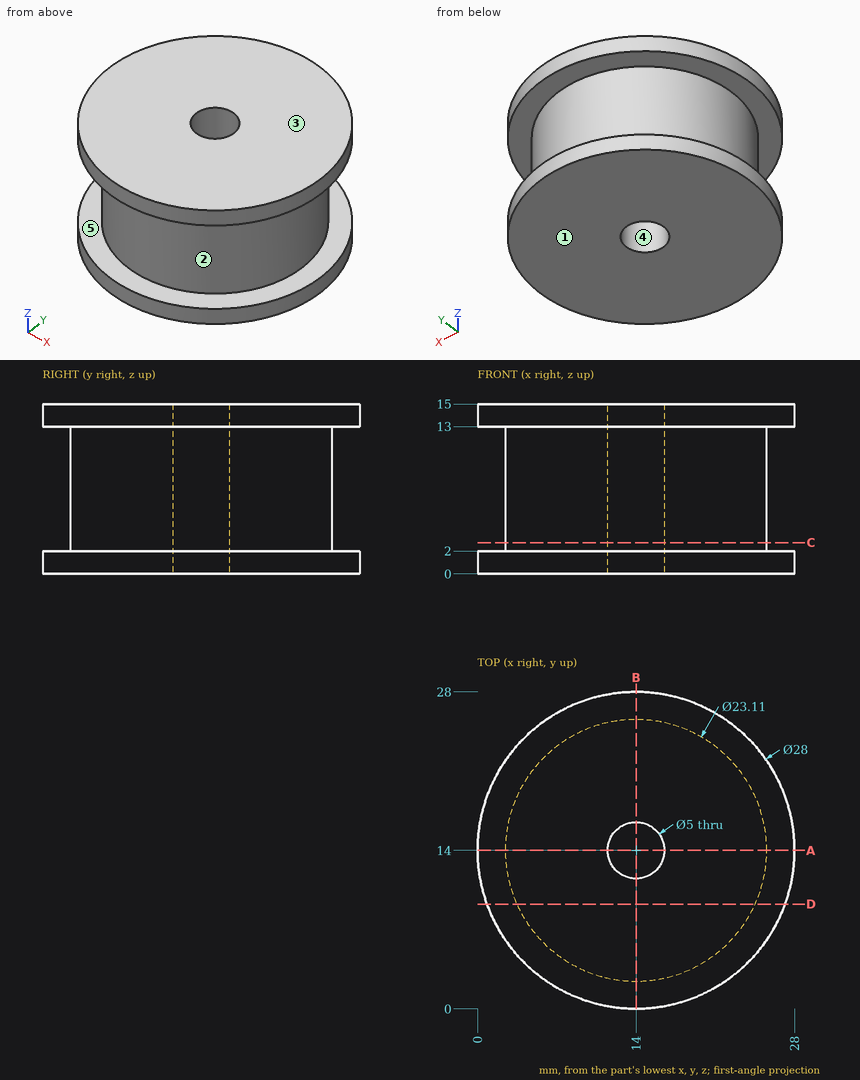
Design review of the part shown in the three views and the two pictorial views. Dimensions are in mm from the part's minimum x, y and z. A direction names the side the tool comes from. Give positions to 0.01 mm unless a question says otherwise; leave off trailing zeros. Write each loop counter-clockwise with the first axis right and the second up, starting at its lowest first coordinate (ties: lowest second). Pieces come first, ordered by that corner, then holes. Notation, with made-up numbers: M -25.75,-38 L 24.25,-38 A10 cw 24.25,-34 Z; hole C 14.25,-18 d11. An arc over 180 degrees is marked long. One line per item, written item: value.
1) Take a section at C-C, the plane z = 2.75. Write out the cut boundary in (x, y) (3 decimals), then the cut area to 3 significant figures.
Results are:
outline: C 14,14 d23.11; hole C 14,14 d5
area: 400 mm²
2) For P1, Ø6, axis at x = 21.5, z = 2.5, coming from the -Y side; P2, Ø3, axis at x = 14, y = 14, coming from the -Z side; P3, Ø1, axis at y = 15.5, z = 13, coming from the -X side; P4, Ø2, axis at y = 13, z = 8, coming from the +X side (3 decimals), all flat-tipped, find the tip position at first contact; note any pin that passes through.
Results are:
P1: stops at y = 0.76
P2: passes through
P3: stops at x = 0.04
P4: stops at x = 25.555
3) For the marked faces 4 and 5, list the 3-axis set-ups (+Z, -Z, +X, -X, +Y, -Y) from which the entire face can be reached by the end or side of a thin tool; tool diameter is ignored.
Results are:
face 4: +Z, -Z
face 5: none
4) The part is to be moulded in two halves that separate along Z. For the marked faces 1, 2 and 3, say which applies: +Z half, -Z half, draft (parallel to the pull), parting line (faces both ways), or undercut.
Results are:
face 1: -Z half
face 2: undercut
face 3: +Z half
5) Take a section at D-D, the plane y = 9.25. Write out the cut boundary in (x, z), then the cut area to 3 significant figures.
Results are:
outline: M 0.83,0 L 27.17,0 L 27.17,2 L 24.53,2 L 24.53,13 L 27.17,13 L 27.17,15 L 0.83,15 L 0.83,13 L 3.47,13 L 3.47,2 L 0.83,2 Z
area: 337 mm²
6) For line 1 (Z direction, x = 8.5, y = 24.5); line 2 (Y direction, x = 14, z = 7.5) (3 decimals); line 3 (X direction, y = 1, z = 1.75), list the stretches that pass through material, from the lowest coordinate up. Write a range as from..to.
Results are:
line 1: z = 0..2, 13..15
line 2: y = 2.445..11.5, 16.5..25.555
line 3: x = 8.8..19.2
7) Take a section at A-A, the plane y = 14. Write out the cut boundary in (x, z) (3 decimals).
Results are:
outline: M 0,0 L 11.5,0 L 11.5,15 L 0,15 L 0,13 L 2.445,13 L 2.445,2 L 0,2 Z; M 16.5,0 L 28,0 L 28,2 L 25.555,2 L 25.555,13 L 28,13 L 28,15 L 16.5,15 Z
